Geometry check sheet. Reference: the model listing, model coordinates, mm. A direction names the side the tool comes from. Give positions to 0.01 mm unless a question says otherwise; leave off trailing zeros. Write each loop counter-clockwise with the first axis right and the second up, starting at its lowest first coordinate (ties: lowest second). Pieces come first, ordered by that corner, then holes.
(1) Thickness scan on line 1 along X through (y, z) = (5.25, -279.5); line 2 along Z through (x, y) = (-60.5, 2.25); line 3 along Z through (x, y) = (7, 18.5). Record the ranges inside material, lowest first.
(2) Cross-section at B-B (z = -18). Record the boundary of the cut face in (x, y), and give its area (3 significant figures).
(3) Depth check by flat-ended pin: P1, Ø2, axis at x = 102.5, z = 22.5, coming from the -Y side; P2, Ø5, axis at x = 15, y = 6.5, coming from the +Z side; P3, Ø2, axis at x = 19.5, y = 14, coming from the +Z side. Enter the tip coordinate at first touch or a pass-through.
(4) Cross-section at C-C (y = 4.25). Record the boundary of the cut face in (x, z), and give its area (3 significant figures).
(5) Mould release check, pull along Z, two halves, no side actions. Record for faces 1 (the flat face through (-102, 19.53, -121)), 2 (the flat face through (-7.427, 10, 19)), 3 (the flat face through (-79, 10, 173.337)): +Z half, -Z half, draft (parallel to the pull), parting line (faces both ways), or undercut.
(6) Cross-section at A-A (x = 93.5). Record the boundary of the cut face in (y, z).
(7) Tool access check on faces 4 (the flat face through (-157.427, 10, -113)), 5 (the flat face through (-9, 9.53, 133)), 6 (the flat face through (-45, 10, -11.663)). Record the directions out of +Z, -Z, +X, -X, +Y, -Y that give a thin tool (end or side, any length) a straight path to the whole face; none if there is none.
```python
from build123d import *

# Parameters (mm, degrees)
SKETCH1_W                      = 345
SKETCH1_H                      = 580
BOSS_EXTRUDE1_DEPTH            = 19.53
CUT_EXTRUDE1_REACH             = 450.263
SKETCH2_W                      = 215
SKETCH2_H                      = 325
CUT_EXTRUDE1_DIRECTION_2_DEPTH = 449.2627239
SKETCH3_W                      = 45
SKETCH3_H                      = 60
CUT_EXTRUDE2_DEPTH             = 19.53
SKETCH4_W                      = 105
SKETCH4_H                      = 80
CUT_EXTRUDE3_DEPTH             = 10
SKETCH5_W                      = 25
SKETCH5_H                      = 60
CUT_EXTRUDE4_DEPTH             = 10


with BuildPart() as part:
    # Sketch1 → Boss-Extrude1 (new body)
    with BuildSketch(Plane(origin=(0, 0, 0), x_dir=(1, 0, 0), z_dir=(0, 1, 0))):
        with Locations((15.072815534, 116.662621359)):
            Rectangle(SKETCH1_W, SKETCH1_H)
    extrude(amount=BOSS_EXTRUDE1_DEPTH)

    # Sketch2 → Cut-Extrude1 (cut, up to next)
    with BuildSketch(Plane(origin=(0, 19.53, 0), x_dir=(1, 0, 0), z_dir=(0, 1, 0)), mode=Mode.PRIVATE) as cut_extrude1_sk1:
        with Locations((25.072815534, 174.162621359)):
            Rectangle(SKETCH2_W, SKETCH2_H)
    cut_extrude1_tool1 = extrude(cut_extrude1_sk1.sketch, amount=-CUT_EXTRUDE1_REACH, mode=Mode.PRIVATE) & part.part
    add(cut_extrude1_tool1.solids().sort_by_distance((25.072816, 19.53, -174.162621))[0], mode=Mode.SUBTRACT)

    # Sketch2 → Cut-Extrude1 direction 2 (cut)
    with BuildSketch(Plane(origin=(0, 19.53, 0), x_dir=(1, 0, 0), z_dir=(0, 1, 0))):
        with Locations((25.072815534, 174.162621359)):
            Rectangle(SKETCH2_W, SKETCH2_H)
    extrude(amount=CUT_EXTRUDE1_DIRECTION_2_DEPTH, mode=Mode.SUBTRACT)

    # Sketch3 → Cut-Extrude2 (cut)
    with BuildSketch(Plane(origin=(0, 19.53, 0), x_dir=(1, 0, 0), z_dir=(0, 1, 0))):
        with Locations((15.072815534, -18.337378641)):
            Rectangle(SKETCH3_W, SKETCH3_H)
    extrude(amount=-CUT_EXTRUDE2_DEPTH, mode=Mode.SUBTRACT)

    # Sketch4 → Cut-Extrude3 (cut)
    with BuildSketch(Plane(origin=(0, 19.53, 0), x_dir=(1, 0, 0), z_dir=(0, 1, 0))):
        with Locations((15.072815534, -133.337378641)):
            Rectangle(SKETCH4_W, SKETCH4_H)
    extrude(amount=-CUT_EXTRUDE3_DEPTH, mode=Mode.SUBTRACT)

    # Sketch5 → Cut-Extrude4 (cut)
    with BuildSketch(Plane(origin=(0, 9.53, 0), x_dir=(1, 0, 0), z_dir=(0, 1, 0))):
        with Locations((15.072815534, -143.337378641)):
            Rectangle(SKETCH5_W, SKETCH5_H)
    extrude(amount=-CUT_EXTRUDE4_DEPTH, mode=Mode.SUBTRACT)


solid = part.part
```
Reply:
1. line 1: x = -157.43 to -82.43, 132.57 to 187.57
1. line 2: z = -406.66 to -336.66, -11.66 to 173.34
1. line 3: z = -406.66 to -336.66, 48.34 to 93.34
2. outline: (-157.43, 0) - (-82.43, 0) - (-82.43, 19.53) - (-157.43, 19.53) - close; (132.57, 0) - (187.57, 0) - (187.57, 19.53) - (132.57, 19.53) - close
2. area: 2,540 mm2
3. P1: stops at y = 0
3. P2: stops at z = 113.34
3. P3: stops at z = 93.34
4. outline: (-157.43, -406.66) - (187.57, -406.66) - (187.57, 173.34) - (27.57, 173.34) - (27.57, 113.34) - (2.57, 113.34) - (2.57, 173.34) - (-157.43, 173.34) - close; hole (-82.43, -336.66) - (132.57, -336.66) - (132.57, -11.66) - (37.57, -11.66) - (37.57, 48.34) - (-7.43, 48.34) - (-7.43, -11.66) - (-82.43, -11.66) - close
4. area: 126,000 mm2
5. face 1: draft
5. face 2: undercut
5. face 3: +Z half
6. outline: (0, -406.66) - (19.53, -406.66) - (19.53, -336.66) - (0, -336.66) - close; (0, -11.66) - (19.53, -11.66) - (19.53, 173.34) - (0, 173.34) - close
7. face 4: +Z, -Z, -X, +Y, -Y
7. face 5: +Z, +Y
7. face 6: +Y, -Y
